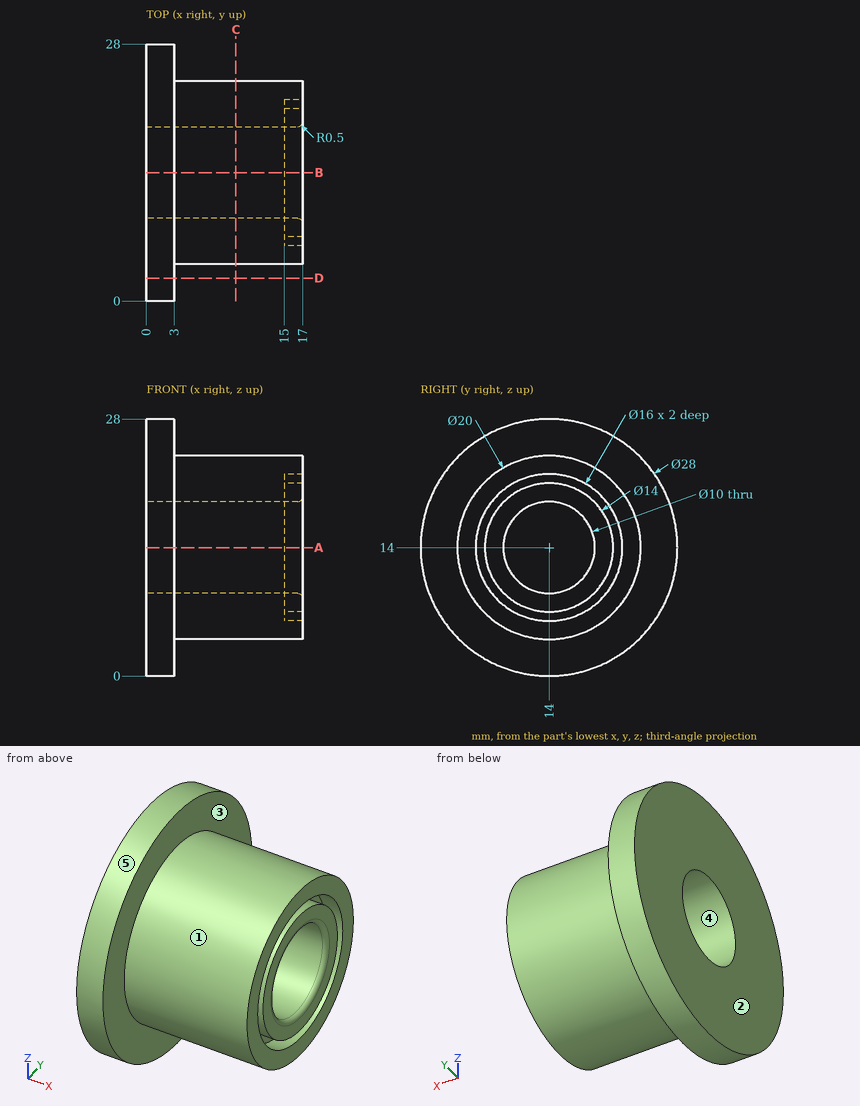
Could you check a few things on this drawing? It's one solid part, dimensions in mm from its lowest x, y, z. A direction names the side the tool comes from. Give positions to 0.01 mm unless a question says otherwise; leave off trailing zeros. Loops run counter-clockwise (first coordinate to the right, second up) from the corner with the lowest first, then second, coordinate; pieces in that order, holes last. Notation, with made-up numbers: M 85.25,45.5 L 142.25,45.5 A24 cw 142.25,83.5 Z; hole C 55.5,-29 d4. An arc over 180 degrees is marked long. Answer as a JSON object with one key per item and string values.
Q1. Suppose I cut it at D-D, the plane y = 2.5. List the corners of the cut face in (x, z) for me, plus the area to 3 significant figures.
Values found:
{"outline": "M 0,6.02 L 3,6.02 L 3,21.98 L 0,21.98 Z", "area": "47.9 mm²"}
Q2. If we mould it in two halves opening along Y, with no side actions, what happens to the marked faces 3, 4 and 5? For each: pulls with the +Y half, pulls with the -Y half, needs draft (parallel to the pull), parting line crosses it, or undercut.
Values found:
{"face 3": "needs draft", "face 4": "undercut", "face 5": "parting line crosses it"}
Q3. For the marked faces 1 and 2, which set-ups out of +Z, -Z, +X, -X, +Y, -Y let a thin tool reach every point of the face, with its end or its side?
Values found:
{"face 1": "+X", "face 2": "+Z, -Z, -X, +Y, -Y"}
Q4. If I drill on probe 1 along Z at (x, y) = (15.75, 14); probe 2 along Y at (x, z) = (16.25, 8.5); probe 3 along Z at (x, y) = (3.75, 14), over which ranges is the centre line in solid material (lowest first)? Write a range as [from, to].
Values found:
{"probe 1": "z = [4, 6], [7, 9], [19, 21], [22, 24]", "probe 2": "y = [5.65, 8.19], [9.67, 18.33], [19.81, 22.35]", "probe 3": "z = [4, 9], [19, 24]"}
Q5. Suppose I cut it at A-A, the plane z = 14. List the corners of the cut face in (x, y) for me, plus the area to 3 significant figures.
Values found:
{"outline": "M 0,0 L 3,0 L 3,4 L 17,4 L 17,6 L 15,6 L 15,7 L 17,7 L 17,8.5 A0.5 ccw 16.5,9 L 0,9 Z; M 0,19 L 16.5,19 A0.5 ccw 17,19.5 L 17,21 L 15,21 L 15,22 L 17,22 L 17,24 L 3,24 L 3,28 L 0,28 Z", "area": "190 mm²"}
Q6. Suppose I cut it at C-C, the plane x = 9.75. List the corners of the cut face in (y, z) for me.
Values found:
{"outline": "C 14,14 d20; hole C 14,14 d10"}
Q7. For P1, Ø10, axis at x = 8.5, y = 22, coming from the -Z side; P2, Ø2, axis at x = 11.5, y = 22.5, coming from the -Z side; P3, Ø5, axis at x = 13.5, z = 3.5, coming from the +Y side, each with a flat end and sliding along its axis, tell me the tip position at first contact or that it passes through.
Values found:
{"P1": "stops at z = 4.46", "P2": "stops at z = 7.39", "P3": "stops at y = 20"}
